Could you check a few things on this drawing? It's one solid part, dimensions in mm from its lowest x, y, z. A direction names the side the tool comes from. Give positions to 0.01 mm unless a question says otherwise; leave off trailing zeros. Loops run counter-clockwise (first coordinate to the right, second up) from the corner with the lowest first, then second, coordinate; pieces in that order, holes last.
Q1. Thinking about a two-plate mould opening in Y: for the marked faces 1, 2, 3 and 4, which applies, pulls with the +Y half, pulls with the -Y half, needs draft (parallel to the pull), parting line crosses it, or undercut?
Q2. For the marked faces 5, 6 and 7, which set-ups out of +Z, -Z, +X, -X, +Y, -Y let a thin tool reach every point of the face, with its end or its side?
Q3. I'm going to push flat-ended pins straight in: P1, Ø6, axis at x = 12.5, z = 24.5, coming from the -Y side; P2, Ø2, axis at y = 7, z = 34.5, coming from the +X side; P3, Ø5, axis at x = 13, z = 11.5, coming from the -Y side; P4, Ø12, axis at x = 12, z = 8, coming from the +Y side. Where does each tip first touch, or does it pass through?
Q4. Suppose I cut it at D-D (x = 16.5). List the corners of the cut face in (y, z) for me.
Q5. Suppose I cut it at B-B (z = 13.5). List the corners of the cut face in (x, y) for me, and give its area (3 significant figures).
Q6. Suppose I cut it at C-C (x = 10.75). List the corners of the cut face in (y, z) for me.
Q7. I need wall thicknesses on probe 1 along Y at (x, z) = (12.85, 8); probe 2 along X at (y, z) = (17, 17); probe 3 along Z at (x, y) = (3.25, 13.75). Which ranges of each line are inside material? Lowest first, please.
Q8. Suppose I cut it at A-A (y = 14). List the corners of the cut face in (x, z) for me.
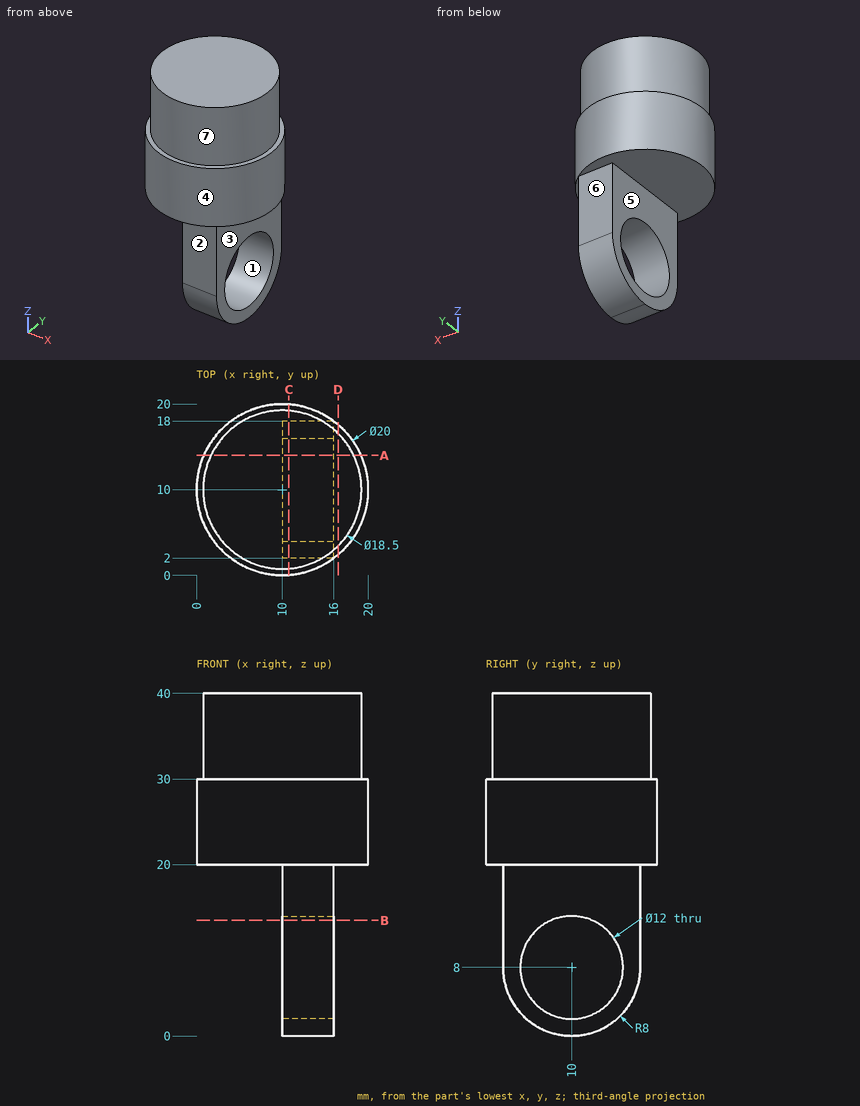
Solutions:
1. face 1: undercut
1. face 2: pulls with the -Y half
1. face 3: needs draft
1. face 4: parting line crosses it
2. face 5: -Z, -X, +Y, -Y
2. face 6: -Z, +X, -X, +Y
2. face 7: +Z
3. P1: stops at y = 0
3. P2: stops at x = 19.03
3. P3: stops at y = 2
3. P4: stops at y = 18
4. outline: (2.4, 20) - (17.6, 20) - (17.6, 30) - (16.58, 30) - (16.58, 40) - (3.42, 40) - (3.42, 30) - (2.4, 30) - close
5. outline: (10, 2) - (16, 2) - (16, 7.6) - (10, 7.6) - close; (10, 12.4) - (16, 12.4) - (16, 18) - (10, 18) - close
5. area: 67.2 mm2
6. outline: (0.03, 20) - (2, 20) - (2, 8) arc R8 ccw to (18, 8) - (18, 20) - (19.97, 20) - (19.97, 30) - (19.22, 30) - (19.22, 40) - (0.78, 40) - (0.78, 30) - (0.03, 30) - close; hole circle Ø12 at (10, 8)
7. probe 1: y = 2 to 4, 16 to 18
7. probe 2: x = 10 to 16
7. probe 3: z = 20 to 40
8. outline: (0.83, 20) - (10, 20) - (10, 12.47) - (16, 12.47) - (16, 20) - (19.17, 20) - (19.17, 30) - (18.34, 30) - (18.34, 40) - (1.66, 40) - (1.66, 30) - (0.83, 30) - close; (10, 1.07) - (16, 1.07) - (16, 3.53) - (10, 3.53) - close
